Check sheet for the modelled part. Datum: model origin and axes. Units: mm. A direction names the side the tool comes from. Give positions to 0.01 mm unless a question says otherwise; leave off trailing zeros. Loops run counter-clockwise (first coordinate to the right, second up) from the corner with the lowest first, then second, coordinate; pieces in that order, holes last. Notation, with made-up numbers: (38.5, -2.75) - (48.5, -2.75) arc R25 cw to (48.5, 11.25) - close; hole circle Ø6 at (32.25, 61.25). An arc over 180 degrees is marked (long way). Use CSV: the item, a comma, the result in double quotes.
from build123d import *

# Parameters (mm, degrees)
F0_W     = 152.4
F0_H     = 101.6
F1_DEPTH = 152.4
F2_W     = 152.4
F2_H     = 0.8561833287
F3_DEPTH = 76.2
F4_R     = 12.7


with BuildPart() as f1:
    # F0 (on Front) → F1 (new body)
    with BuildSketch(Plane.XZ):
        with BuildLine():
            Line((0, 0), (0, -254))
            Line((0, -254), (609.6, -254))
            Line((609.6, -254), (609.6, 0))
            ThreePointArc((609.6, 0), (515.2777766961, 30.2643447869), (456.1725186703, 109.7576202765))
            ThreePointArc((456.1725186703, 109.7576202765), (304.8, 218.0451791971), (153.4274813297, 109.7576202765))
            ThreePointArc((153.4274813297, 109.7576202765), (94.3222233039, 30.2643447869), (0, 0))
        make_face()
        with Locations((304.8, 58.1014369479)):
            Rectangle(F0_W, F0_H, mode=Mode.SUBTRACT)
    extrude(amount=F1_DEPTH)

    # F2 (on face) → F3 (cut)
    with BuildSketch(Plane.XZ.offset(152.4)):
        with Locations((304.8, 109.3295286122)):
            Rectangle(F2_W, F2_H)
    extrude(amount=-F3_DEPTH, mode=Mode.SUBTRACT)

    # F4
    f4_edges = [f1.edges().sort_by_distance(p)[0] for p in [
        (609.6, -76.2, 0),
        (0, -76.2, 0),
        (515.277777, -152.4, 30.264345),
        (304.8, -152.4, 218.045179),
        (304.8, 0, 218.045179),
        (515.277777, 0, 30.264345),
        (609.6, -152.4, -127),
        (609.6, 0, -127),
        (0, -152.4, -127),
        (0, 0, -127),
    ]]
    fillet(f4_edges, radius=F4_R)


solid = f1.part
1. Scan lines: line 1 along X through (y, z) = (-125, 81); line 2 along Y through (x, z) = (136.5, 55); line 3 along X through (y, z) = (-8, 25). Record each from-to range of solid material in increasing order.
Completed:
line 1,"x = 140.36 to 228.6, 381 to 469.24"
line 2,"y = -152.33 to -0.07"
line 3,"x = 88.17 to 228.6, 381 to 521.43"
2. Release check for a two-part mould opening along Z. For faces 1 (the face through (304, -115, 109.758)), 2 (the face through (3.62, -148.58, -134.81)), 3 (the face through (228.6, -75, 58)), 4 (the face through (606.11, -77.089, -3.493)) record: released by +Z, released by -Z, zero draft, split by the parting line, or undercut.
Completed:
face 1,"undercut"
face 2,"zero draft"
face 3,"undercut"
face 4,"released by +Z"
3. Set-up check for faces 5 (the face through (3.3, -77.1, -3.7)), 6 (the face through (304, -75, 7.301)): record each of +Z, -Z, +X, -X, +Y, -Y from which the full face is reachable in a straight line by a thin tool's end or side.
Completed:
face 5,"+Z, -X, +Y, -Y"
face 6,"+Y, -Y"
4. Sectioned sample at B-B, the plane y = -93.5. Record the boundary of the cut face in (x, z).
Completed:
outline,"(0, -254) - (609.6, -254) - (609.6, -12.24) arc R12.7 ccw to (597.82, 0.43) arc R162.12 cw to (456.17, 109.76) arc R159.94 ccw to (153.43, 109.76) arc R162.12 cw to (11.78, 0.43) arc R12.7 ccw to (0, -12.24) - close; hole (228.6, 7.3) - (381, 7.3) - (381, 109.76) - (228.6, 109.76) - close"
5. Go/stop test with flat-tipped pins: pin 1 Ø3 at (y, z) = (-119, 143.5) entering from -X; pin 2 Ø4 at (x, y) = (148, -126) entering from +Z; pin 3 Ø4 at (x, y) = (116, -116) entering from +Z. Record where each tip stops, or that it passes through.
Completed:
pin 1,"stops at x = 168.63"
pin 2,"stops at z = 100.62"
pin 3,"stops at z = 50.95"
6. Sectioned sample at A-A, the plane y = -30.5. Record the boundary of the cut face in (x, z).
Completed:
outline,"(0, -254) - (609.6, -254) - (609.6, -12.24) arc R12.7 ccw to (597.82, 0.43) arc R162.12 cw to (456.17, 109.76) arc R159.94 ccw to (153.43, 109.76) arc R162.12 cw to (11.78, 0.43) arc R12.7 ccw to (0, -12.24) - close; hole (228.6, 7.3) - (381, 7.3) - (381, 108.9) - (228.6, 108.9) - close"
